Here's the drawing with two shaded views (mm, measured from the low corner). I have some questions. A direction names the side the tool comes from. Coordinates: 2 decimals unless noted, no trailing zeros. Write each loop counter-clockwise with the first axis right and the second up, starting at its lowest first coordinate (ties: lowest second). Pieces come first, ordered by that corner, then holes.
Item 1: If we section it at D-D (y = 2.5): Please give me the cut outline in (x, z), then the cut area to 3 significant figures.
Item 2: If I drill on line 1 (Y direction, x = 2, z = 3); line 2 (Y direction, x = 25, z = 6.5); line 3 (Z direction, x = 7, y = 12.75), over which ranges is the centre line in solid material (lowest first)?
Item 3: If we section it at B-B (z = 2.5): Please give me the cut outline in (x, y), then the cut area to 3 significant figures.
Item 4: If we section it at C-C (x = 14): Please give me the cut outline in (y, z).
Item 5: We'd pull the mould along Y, two halves only. Please class the marked faces 3, 4, 5 and 6: +Y half, -Y half, draft (parallel to the pull), parting line (faces both ways), or undercut.
Item 6: For the marked faces 1 and 2, which set-ups out of +Z, -Z, +X, -X, +Y, -Y let a thin tool reach every point of the face, with its end or its side?
Item 7: I'm going to push flat-ended pins straight in: pin 1 Ø1.8 at (x, y) = (29, 14) entering from -Z; pin 2 Ø5 at (x, y) = (10.5, 12.5) entering from +Z. Where does each tip first touch, or does it pass through?
Item 8: If we section it at A-A (z = 7.25): Please give me the cut outline in (x, y), then the cut area to 3 significant figures.
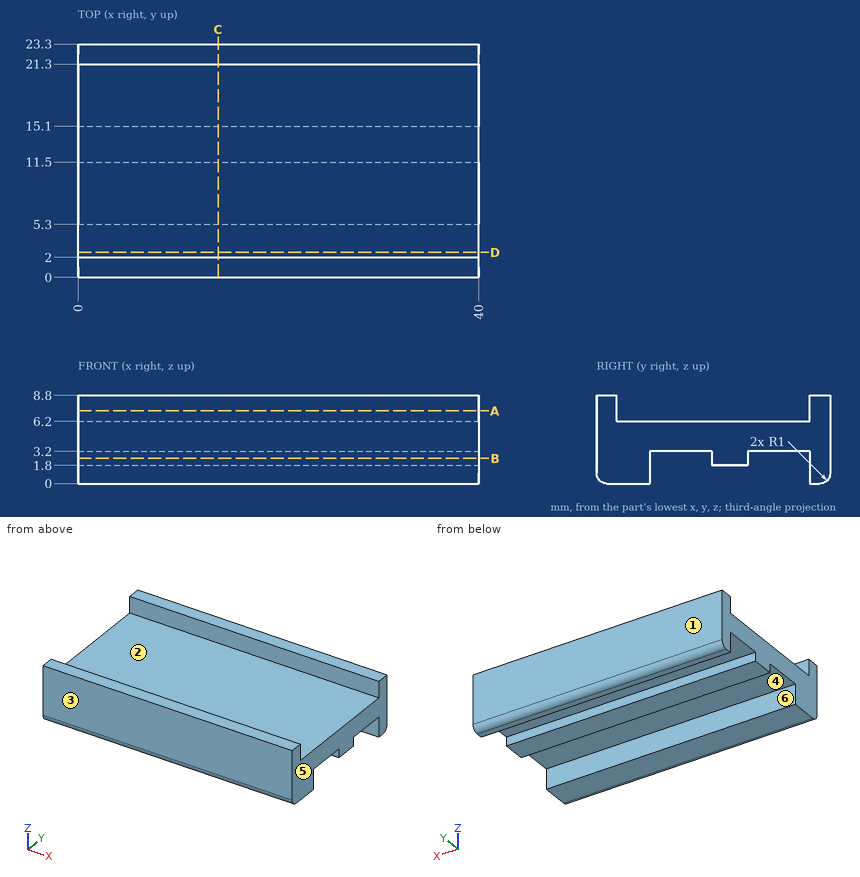
Answer list:
1. outline: (0, 0) - (40, 0) - (40, 6.2) - (0, 6.2) - close
1. area: 248 mm2
2. line 1: y = 0 to 5.3, 11.5 to 15.1, 21.3 to 23.3
2. line 2: y = 0 to 2, 21.3 to 23.3
2. line 3: z = 1.8 to 6.2
3. outline: (0, 0) - (40, 0) - (40, 5.3) - (0, 5.3) - close; (0, 11.5) - (40, 11.5) - (40, 15.1) - (0, 15.1) - close; (0, 21.3) - (40, 21.3) - (40, 23.3) - (0, 23.3) - close
3. area: 436 mm2
4. outline: (0, 1) arc R1 ccw to (1, 0) - (5.3, 0) - (5.3, 3.2) - (11.5, 3.2) - (11.5, 1.8) - (15.1, 1.8) - (15.1, 3.2) - (21.3, 3.2) - (21.3, 0) - (22.3, 0) arc R1 ccw to (23.3, 1) - (23.3, 8.8) - (21.3, 8.8) - (21.3, 6.2) - (2, 6.2) - (2, 8.8) - (0, 8.8) - close
5. face 3: -Y half
5. face 4: undercut
5. face 5: draft
5. face 6: undercut
6. face 1: +Z, -Z, +X, -X, +Y
6. face 2: +Z, +X, -X
7. pin 1: stops at z = 1.8
7. pin 2: stops at z = 6.2
8. outline: (0, 0) - (40, 0) - (40, 2) - (0, 2) - close; (0, 21.3) - (40, 21.3) - (40, 23.3) - (0, 23.3) - close
8. area: 160 mm2
